Geometry check sheet. Reference: drawing and pictorial views, mm from the part's lowest x, y, z. A direction names the side the tool comes from. Round coordinates to 2 decimals unless told otherwise and drop trailing zeros. Loops run counter-clockwise (first coordinate to the right, second up) from the corner with the lowest first, then second, coordinate; pieces in that order, holes last. Notation, with made-up numbers: M 81,15 L 88,15 A18 cw 88,27 Z; hole C -12,62.5 d5. An arc over 180 degrees is marked long. One line per question, with ' | ' between items. Start each with the question number.
(1) Draft check along Z on the marked faces 1, 2 and 3. Enter one of: +Z half, -Z half, draft (parallel to the pull), parting line (faces both ways), or undercut.
(2) Go/stop test with flat-tipped pins: P1, Ø4, axis at y = 9.5, z = 50, coming from the -X side; P2, Ø15, axis at x = 79, z = 59.5, coming from the -Y side; P3, Ø10, axis at x = 81.5, y = 14.5, coming from the -Z side. Record where each tip stops, or that it passes through.
(3) Section check C-C (x = 62). Record the boundary of the cut face in (y, z).
(4) Thickness scan on probe 1 along Z at (x, y) = (9.5, 4) (1 decimal); probe 2 along X at (y, z) = (24.5, 130.5); probe 3 along X at (y, z) = (20.5, 171.5). Record the ranges inside material, lowest first. Write a range as [from, to].
(5) Tool access check on the marked faces 4 and 5. Record the directions out of +Z, -Z, +X, -X, +Y, -Y that give a thin tool (end or side, any length) a straight path to the whole face; none if there is none.
(6) Section check B-B (y = 15.25). Record the boundary of the cut face in (x, z) (1 decimal), and give its area (3 significant figures).
(7) Section check A-A (z = 50.5). Record the boundary of the cut face in (x, y) (1 decimal).
(8) Section check D-D (z = 128.5). Record the boundary of the cut face in (x, y), and give its area (3 significant figures).
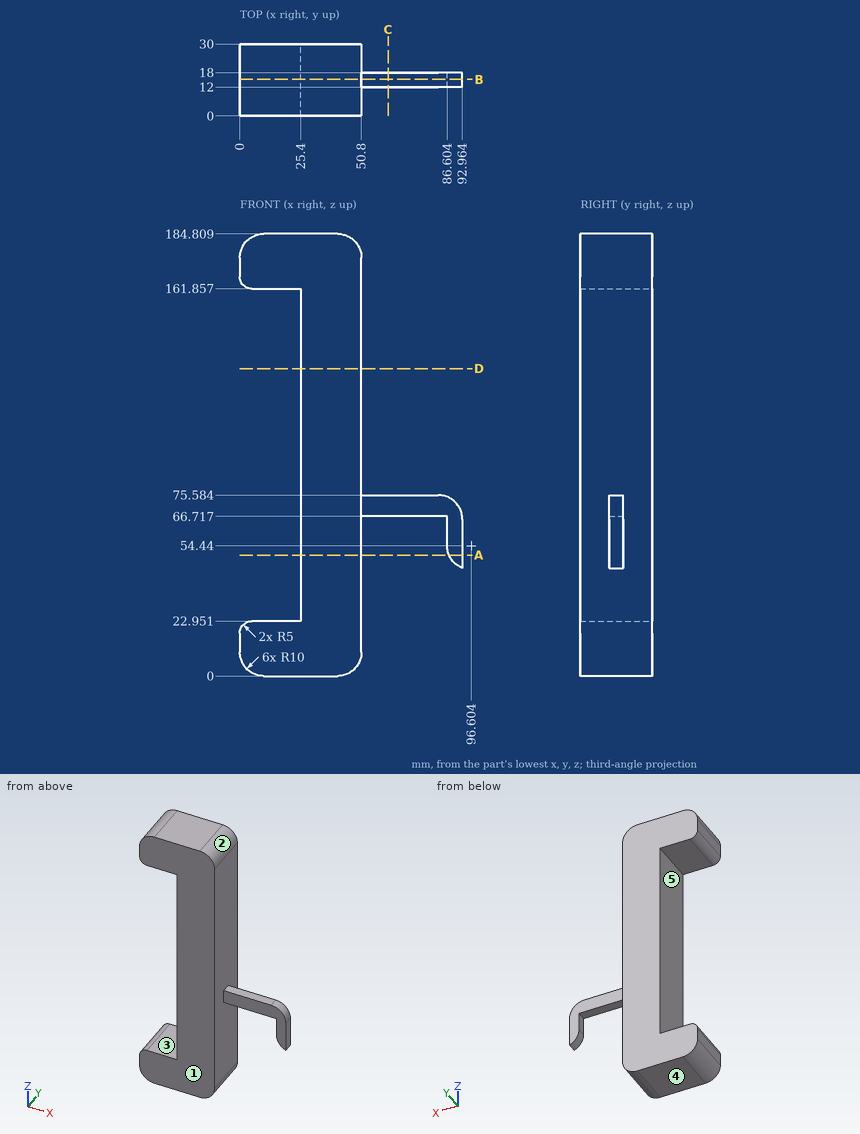
The answers:
1) face 1: draft | face 2: +Z half | face 3: undercut
2) P1: x = 25.4 | P2: y = 12 | P3: z = 66.72
3) outline: M 12,66.72 L 18,66.72 L 18,75.58 L 12,75.58 Z
4) probe 1: [0, 23], [161.9, 184.8] | probe 2: [25.4, 50.8] | probe 3: [0, 50.8]
5) face 4: -Z, +X, -X, +Y, -Y | face 5: -X, +Y, -Y
6) outline: M 0,10 A10 ccw 10,0 L 40.8,0 A10 ccw 50.8,10 L 50.8,66.7 L 86.6,66.7 L 86.6,54.4 A10 ccw 93,45.1 L 93,65.6 A10 ccw 83,75.6 L 50.8,75.6 L 50.8,174.8 A10 ccw 40.8,184.8 L 10,184.8 A10 ccw 0,174.8 L 0,166.9 A5 ccw 5,161.9 L 25.4,161.9 L 25.4,23 L 5,23 A5 ccw 0,18 Z | area: 6,240 mm²
7) outline: M 25.4,0 L 50.8,0 L 50.8,30 L 25.4,30 Z; M 87.4,12 L 93,12 L 93,18 L 87.4,18 Z
8) outline: M 25.4,0 L 50.8,0 L 50.8,30 L 25.4,30 Z | area: 762 mm²
